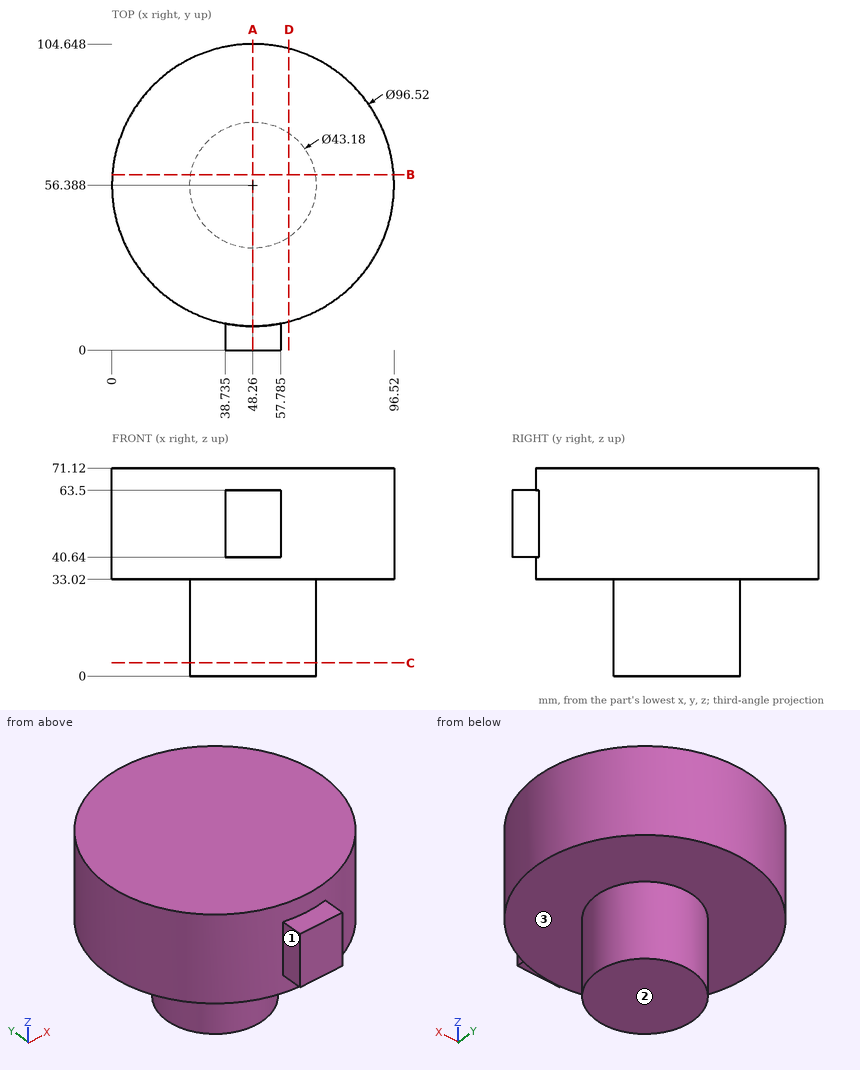
Source: three-view drawing plus pictorial views. Frame: mm from the lowest corner of the part. A direction names the side the tool comes from. Coordinates: 2 decimals unless noted, no trailing zeros. Write each loop counter-clockwise with the first axis right and the second up, starting at its lowest first coordinate (ties: lowest second). Pieces come first, ordered by that corner, then holes. Notation, with made-up numbers: (-17.5, -15.75) - (18.5, -15.75) arc R34 ccw to (18.5, 21.25) - close; hole circle Ø6 at (-10, 69.5). An arc over 180 degrees is marked (long way). Answer as a JSON object with one key per item and string values.
Q1. Set-up query: the marked faces 1, 2 and 3. Return all of +Z, -Z, +X, -X, +Y, -Y with unobstructed straight access to the full face (end or side cutting, diameter ignored); none if empty.
Ans:
{"face 1": "+Z, -Z, -X, -Y", "face 2": "-Z, +X, -X, +Y, -Y", "face 3": "-Z"}
Q2. Section query C-C, the plane z = 4.5. Output: boundary loops of the cut face in (x, y).
Ans:
{"outline": "circle Ø43.18 at (48.26, 56.39)"}
Q3. Section query D-D, the plane x = 60.5. Output: boundary loops of the cut face in (y, z).
Ans:
{"outline": "(9.71, 33.02) - (38.6, 33.02) - (38.6, 0) - (74.17, 0) - (74.17, 33.02) - (103.07, 33.02) - (103.07, 71.12) - (9.71, 71.12) - close"}
Q4. Section query A-A, the plane x = 48.26. Output: boundary loops of the cut face in (y, z), plus the area to 3 significant figures.
Ans:
{"outline": "(0, 40.64) - (8.13, 40.64) - (8.13, 33.02) - (34.8, 33.02) - (34.8, 0) - (77.98, 0) - (77.98, 33.02) - (104.65, 33.02) - (104.65, 71.12) - (8.13, 71.12) - (8.13, 63.5) - (0, 63.5) - close", "area": "5,290 mm2"}
Q5. Section query B-B, the plane y = 60. Output: boundary loops of the cut face in (x, z), plus the area to 3 significant figures.
Ans:
{"outline": "(0.14, 33.02) - (26.97, 33.02) - (26.97, 0) - (69.55, 0) - (69.55, 33.02) - (96.38, 33.02) - (96.38, 71.12) - (0.14, 71.12) - close", "area": "5,070 mm2"}
Q6. Material intervals for line 1 (X direction, y = 37, z = 13.5); line 2 (Z direction, x = 23, y = 29.5); line 3 (Y direction, x = 48.5, z = 29), sorted ascending. Write a range as [from, to].
Ans:
{"line 1": "x = [38.76, 57.76]", "line 2": "z = [33.02, 71.12]", "line 3": "y = [34.8, 77.98]"}
Q7. First-contact query: pin 1 Ø6 at (x, z) = (45, 17) entering from +Y; pin 2 Ø10 at (x, y) = (46, 5.5) entering from -Z; pin 3 Ø4.5 at (y, z) = (4.5, 47) entering from -X (3 decimals). Flat tips, straight axial feed; report the tip coordinate or a pass-through.
Ans:
{"pin 1": "stops at y = 77.98", "pin 2": "stops at z = 33.02", "pin 3": "stops at x = 38.735"}
